Source: CAD feature listing. Evaluate the final solid. Frame: model axes, mm. A direction names the side the tool comes from. Round coordinates to 2 decimals unless told otherwise and drop trailing zeros. Loops run counter-clockwise (first coordinate to the right, second up) from the corner with the lowest first, then second, coordinate; pieces in that order, holes last. Notation, with made-up numbers: M -2,81 L 33,81 A15 ccw 33,101 Z; hole C 55,64.25 d2. An arc over 180 degrees is marked long. Write each question's results on one line, items separated by ' | '. Start each with the question number.
1. Section D-D on y = 2. Output: boundary loops of the cut face in (x, z), and give its area (3 significant figures).
2. Draft query along X for faces 4 (the flat face through (0, 0, 20)), 5 (the flat face through (10, 0, 10)), 6 (the flat face through (-10, 0, 10)), 7 (the flat face through (-8, -7, 10)). Return one class per face: released by +X, released by -X, zero draft, split by the parting line, or undercut.
3. Ray query, line 1 (X direction, y = 6, z = 1); line 2 (Y direction, x = 5, z = 12.25); line 3 (X direction, y = 2.25, z = 18.5). Return the intervals inside material, ascending.
4. Contact query for flat-ended pins moving along their axis: pin 1 Ø6 at (x, z) = (-4, 3.5) entering from +Y; pin 2 Ø3 at (x, z) = (-0.5, 7.5) entering from +Y; pin 3 Ø11 at (x, z) = (0.5, 8.5) entering from -Y. Output: stop coordinate, or through.
5. Section A-A on y = 5.5. Output: boundary loops of the cut face in (x, z), and give its area (3 significant figures).
6. Set-up query: faces 1 (the flat face through (9, -10, 10)), 2 (the flat face through (-8, 7, 10)), 3 (the flat face through (8, -7, 10)). Return all of +Z, -Z, +X, -X, +Y, -Y with unobstructed straight access to the full face (end or side cutting, diameter ignored); none if empty.
7. Section C-C on x = -2.5. Output: boundary loops of the cut face in (y, z), and give its area (3 significant figures).
8. Section B-B on z = 11. Output: boundary loops of the cut face in (x, y), and give its area (3 significant figures).
from build123d import *

# Parameters (mm, degrees)
BOSS_EXTRUDE2_DEPTH = 20
FILLET1_R           = 3
FILLET2_R           = 3


with BuildPart() as part:
    # Sketch2 → Boss-Extrude2 (new body)
    with BuildSketch(Plane.XY):
        Polygon((-10, -10), (-8, -10), (-8, -1.5), (8, -1.5), (8, -10), (10, -10), (10, 10), (8, 10), (8, 1.5), (-8, 1.5), (-8, 10), (-10, 10), align=None)
    extrude(amount=BOSS_EXTRUDE2_DEPTH)

    # Fillet1
    fillet1_edges = [part.edges().sort_by_distance(p)[0] for p in [
        (-8, 1.5, 10),
    ]]
    fillet(fillet1_edges, radius=FILLET1_R)

    # Fillet2
    fillet2_edges = [part.edges().sort_by_distance(p)[0] for p in [
        (8, 1.5, 10),
        (8, -1.5, 10),
        (-8, -1.5, 10),
    ]]
    fillet(fillet2_edges, radius=FILLET2_R)


solid = part.part
Taken from the geometry:
1) outline: M -10,0 L -6.66,0 L -6.66,20 L -10,20 Z; M 6.66,0 L 10,0 L 10,20 L 6.66,20 Z | area: 134 mm^2
2) face 4: zero draft | face 5: released by +X | face 6: released by -X | face 7: undercut
3) line 1: -10 to -8, 8 to 10 | line 2: -1.5 to 1.5 | line 3: -10 to -6.98, 6.98 to 10
4) pin 1: y = 2.26 | pin 2: y = 1.5 | pin 3: y = -1.67
5) outline: M -10,0 L -8,0 L -8,20 L -10,20 Z; M 8,0 L 10,0 L 10,20 L 8,20 Z | area: 80.0 mm^2
6) face 1: +Z, -Z, +X, -X, -Y | face 2: +Z, -Z, +Y | face 3: +Z, -Z, -Y
7) outline: M -1.5,0 L 1.5,0 L 1.5,20 L -1.5,20 Z | area: 60.0 mm^2
8) outline: M -10,-10 L -8,-10 L -8,-4.5 A3 cw -5,-1.5 L 5,-1.5 A3 cw 8,-4.5 L 8,-10 L 10,-10 L 10,10 L 8,10 L 8,4.5 A3 cw 5,1.5 L -5,1.5 A3 cw -8,4.5 L -8,10 L -10,10 Z | area: 136 mm^2
